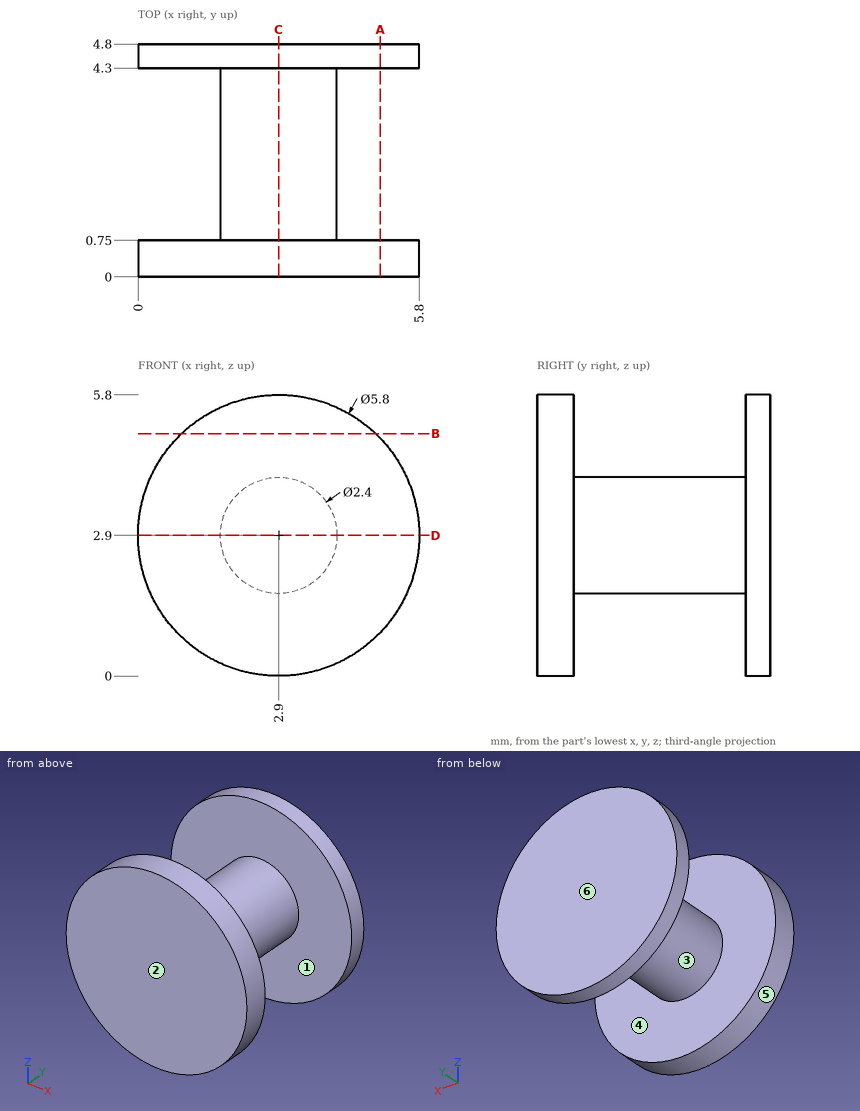
Answer from the drawing. Dimensions are ordinates in mm from the lowest x, y and z of the part. A direction names the side the tool comes from. Coordinates: 2 decimals unless noted, no trailing zeros. Write each loop counter-clockwise with the first axis right and the second up, starting at its lowest first coordinate (ties: lowest second). Pieces come first, ordered by that corner, then holes. Notation, with made-up numbers: M 19,60.5 L 74,60.5 A13 cw 74,65.5 Z; hole C -34.5,37.25 d4. An arc over 180 degrees is marked long. Use one line per item in the form item = value. Start each with the question number.
1. The part is cut by section C-C (x = 2.9). Give the vertices of the cut face in (y, z).
2. The part is cut by section A-A (x = 5). Give the vertices of the cut face in (y, z), plus the area to 3 significant figures.
3. The part is cut by section B-B (z = 5). Give the vertices of the cut face in (x, y), plus the area to 3 significant figures.
4. A tool of negligible diameter and unlimited length cuts with its end or side. For the marked faces 1 and 2, from which of +Z, -Z, +X, -X, +Y, -Y can it reach the whole face along a straight path? Write none if from no direction.
5. The part is cut by section D-D (z = 2.9). Give the vertices of the cut face in (x, y).
6. Straight lines are drawn through the part: probe 1 along Y at (x, z) = (2.05, 4.6); probe 2 along X at (y, z) = (3.25, 2.85); probe 3 along Z at (x, y) = (2.75, 1.5). For each, find the intervals that lie inside material, in ascending order. Write a range as from..to.
7. The mould has two halves that part along Y. Classify the marked faces 3, 4, 5 and 6: released by +Y, released by -Y, zero draft, split by the parting line, or undercut.
Evaluation:
q1.outline = M 0,0 L 0.75,0 L 0.75,1.7 L 4.3,1.7 L 4.3,0 L 4.8,0 L 4.8,5.8 L 4.3,5.8 L 4.3,4.1 L 0.75,4.1 L 0.75,5.8 L 0,5.8 Z
q2.outline = M 0,0.9 L 0.75,0.9 L 0.75,4.9 L 0,4.9 Z; M 4.3,0.9 L 4.8,0.9 L 4.8,4.9 L 4.3,4.9 Z
q2.area = 5.00 mm^2
q3.outline = M 0.9,0 L 4.9,0 L 4.9,0.75 L 0.9,0.75 Z; M 0.9,4.3 L 4.9,4.3 L 4.9,4.8 L 0.9,4.8 Z
q3.area = 5.00 mm^2
q4.face_1 = none
q4.face_2 = +Z, -Z, +X, -X, -Y
q5.outline = M 0,0 L 5.8,0 L 5.8,0.75 L 4.1,0.75 L 4.1,4.3 L 5.8,4.3 L 5.8,4.8 L 0,4.8 L 0,4.3 L 1.7,4.3 L 1.7,0.75 L 0,0.75 Z
q6.probe_1 = 0..0.75, 4.3..4.8
q6.probe_2 = 1.7..4.1
q6.probe_3 = 1.71..4.09
q7.face_3 = undercut
q7.face_4 = undercut
q7.face_5 = zero draft
q7.face_6 = released by +Y
